Can you work these out from the model? Positions are in its coordinate system, mm. A direction names the side the tool comes from. Round coordinates to 2 decimals unless told otherwise and drop trailing zeros. Order: outer loops, then holes, each group sorted by start corner. A loop starts at its lowest first (then second) coordinate and runs counter-clockwise, first axis right, second up. Notation, with made-up numbers: M -38,58.25 L 8,58.25 A19 cw 8,71.25 Z; hole C -36.5,-36.5 d9. An arc over 180 degrees is marked long. One line per question, with ' | ' between items.
```python
from build123d import *

# Parameters (mm, degrees)
SKETCH2_R               = 5
BOSS_EXTRUDE1_DEPTH     = 200
CUT_EXTRUDE1_DEPTH      = 221.996480462
CUT_EXTRUDE1_DEPTH_BACK = 221.996480462
SKETCH3_W               = 142.494389282
SKETCH3_H               = 38.776173082


with BuildPart() as part:
    # Sketch2 → Boss-Extrude1 (new body)
    with BuildSketch(Plane.YZ):
        with BuildLine():
            Line((-63.5, -22.748786417), (-78.5, -22.748786417))
            ThreePointArc((-78.5, -22.748786417), (-82.035533906, -21.284320323), (-83.5, -17.748786417))
            Line((-83.5, -17.748786417), (-83.5, -12.748786417))
            ThreePointArc((-83.5, -12.748786417), (-82.035533906, -9.213252511), (-78.5, -7.748786417))
            Line((-78.5, -7.748786417), (-53.5, -7.748786417))
            Line((-53.5, -7.748786417), (-53.5, 2.251213583))
            Line((-53.5, 2.251213583), (-78.5, 2.251213583))
            ThreePointArc((-78.5, 2.251213583), (-83.151322497, 5.416765702), (-81.913043478, 10.905133973))
            ThreePointArc((-81.913043478, 10.905133973), (0, 43.211044616), (81.913043478, 10.905133973))
            ThreePointArc((81.913043478, 10.905133973), (83.151322497, 5.416765702), (78.5, 2.251213583))
            Line((78.5, 2.251213583), (53.5, 2.251213583))
            Line((53.5, 2.251213583), (53.5, -7.748786417))
            Line((53.5, -7.748786417), (78.5, -7.748786417))
            ThreePointArc((78.5, -7.748786417), (82.035533906, -9.213252511), (83.5, -12.748786417))
            Line((83.5, -12.748786417), (83.5, -17.748786417))
            ThreePointArc((83.5, -17.748786417), (82.035533906, -21.284320323), (78.5, -22.748786417))
            Line((78.5, -22.748786417), (63.5, -22.748786417))
            ThreePointArc((63.5, -22.748786417), (56.754811134, -21.577021257), (50.8, -18.199029134))
            ThreePointArc((50.8, -18.199029134), (0, 0), (-50.8, -18.199029134))
            ThreePointArc((-50.8, -18.199029134), (-56.754811134, -21.577021257), (-63.5, -22.748786417))
        make_face()
        with Locations(Location((0, 31.437967685, 0), (0, 0, 270))):
            Circle(SKETCH2_R, mode=Mode.SUBTRACT)
    extrude(amount=BOSS_EXTRUDE1_DEPTH)

    # Sketch3 → Cut-Extrude1 (cut, two sides: drawn at the far end of the back side and taken through both)
    with BuildSketch(Plane(origin=(0, 0, 0), x_dir=(-1, 0, 0), z_dir=(0, 1, 0)).offset(-CUT_EXTRUDE1_DEPTH_BACK)):
        with Locations((-100, 31.437967685)):
            Rectangle(SKETCH3_W, SKETCH3_H)
    extrude(amount=CUT_EXTRUDE1_DEPTH + CUT_EXTRUDE1_DEPTH_BACK, mode=Mode.SUBTRACT)


solid = part.part
```
(1) If we section it at A-A on y = 0: Please give me the cut outline in (x, z), plus the area to 3 significant figures.
Final values:
outline: M 0,0 L 200,0 L 200,26.44 L 171.25,26.44 L 171.25,12.05 L 28.75,12.05 L 28.75,26.44 L 0,26.44 Z; M 0,36.44 L 28.75,36.44 L 28.75,43.21 L 0,43.21 Z; M 171.25,36.44 L 200,36.44 L 200,43.21 L 171.25,43.21 Z | area: 3,630 mm^2
(2) On a 3-axis mill with a long thin cutter (end or side, diameter ignored), from which of +Z, -Z, +X, -X, +Y, -Y can I reach the whole of each face in a straight line? I mean faces 1 (the flat face through (99, 66, -7.749)), 2 (the flat face through (28.753, -1, 24)), 3 (the cylindrical face through (98.6, -56.664, -21.544)), 4 (the flat face through (99, -53.5, -3)). Say none if no direction works.
Final values:
face 1: +X, -X, +Y | face 2: +Z, +Y, -Y | face 3: -Z, +X, -X | face 4: +X, -X, -Y
(3) Please list where these lines run through material, in increasing order: probe 1 along X at (y, z) = (18, 26); probe 2 along Z at (x, y) = (83, 72); probe 3 along Z at (x, y) = (184.5, 0). Write a range as [from, to].
Final values:
probe 1: [0, 28.75], [171.25, 200] | probe 2: [-22.75, -7.75], [2.25, 12.05] | probe 3: [0, 26.44], [36.44, 43.21]
(4) If we section it at B-B on x = 185: Please give me the cut outline in (y, z), plus the area to 3 significant figures.
Final values:
outline: M -83.5,-17.75 A5 ccw -78.5,-22.75 L -63.5,-22.75 A20 ccw -50.8,-18.2 A80 cw 50.8,-18.2 A20 ccw 63.5,-22.75 L 78.5,-22.75 A5 ccw 83.5,-17.75 L 83.5,-12.75 A5 ccw 78.5,-7.75 L 53.5,-7.75 L 53.5,2.25 L 78.5,2.25 A5 ccw 81.91,10.91 A120 ccw -81.91,10.91 A5 ccw -78.5,2.25 L -53.5,2.25 L -53.5,-7.75 L -78.5,-7.75 A5 ccw -83.5,-12.75 Z; hole C 0,31.44 d10 | area: 6,780 mm^2
(5) If we section it at C-C on z = 31.5: Please give me the cut outline in (x, y).
Final values:
outline: M 0,-51.71 L 28.75,-51.71 L 28.75,-5 L 0,-5 Z; M 0,5 L 28.75,5 L 28.75,51.71 L 0,51.71 Z; M 171.25,-51.71 L 200,-51.71 L 200,-5 L 171.25,-5 Z; M 171.25,5 L 200,5 L 200,51.71 L 171.25,51.71 Z
(6) Will these pins go through, and if not, where does the flat tip stop? pin 1 Ø8 at (x, z) = (118, -2) entering from -Y; pin 2 Ø8 at (x, y) = (134, 56) entering from -Z; pin 3 Ø8 at (x, z) = (79, -0.5) entering from +Y; pin 4 Ø6 at (y, z) = (0, 31.44) entering from +X.
Final values:
pin 1: y = -53.5 | pin 2: z = -22.44 | pin 3: y = 81.81 | pin 4: through
(7) Thinking about a two-plate mould opening in Z: for faces 5 (the flat face through (99, 71, -22.749)), 6 (the cylindrical face through (14.18, 1.5, 26.67)), 7 (the flat face through (101, -1, 12.05)), 8 (the flat face through (99, 83.5, -15)), which applies, released by +Z, released by -Z, zero draft, split by the parting line, or undercut?
Final values:
face 5: released by -Z | face 6: undercut | face 7: released by +Z | face 8: zero draft
(8) If we section it at D-D on y = -69.5: Please give me the cut outline in (x, z).
Final values:
outline: M 0,-22.75 L 200,-22.75 L 200,-7.75 L 0,-7.75 Z; M 0,2.25 L 200,2.25 L 200,21.04 L 171.25,21.04 L 171.25,12.05 L 28.75,12.05 L 28.75,21.04 L 0,21.04 Z
